Here's the drawing with two shaded views (mm, measured from the low corner). I have some questions. Coordinates: 2 decimals unless noted, no trailing zeros. Write each loop counter-clockwise with the first axis right and the second up, starting at its lowest first coordinate (ties: lowest second). Pieces come first, ordered by that corner, then holes. Notation, with made-up numbers: M 8,41 L 67,41 A29 ccw 67,62 Z; hole C 4.5,6.5 d1. An arc over 180 degrees is marked long. Use one line per item in the form item = value. Start each with the question number.
1. I want a section at C-C, the plane y = 17. List the corners of the cut face in (x, z) for me.
2. I want a section at D-D, the plane x = 48. List the corners of the cut face in (y, z) for me, plus the area to 3 significant figures.
3. I want a section at A-A, the plane z = 30. List the corners of the cut face in (x, y) for me.
4. I'm going to push flat-ended pins straight in: pin 1 Ø12 at (y, z) = (5.5, 13.5) entering from +X; pin 2 Ø12 at (y, z) = (16, 35.5) entering from +X; pin 3 Ø6 at (x, z) = (37.5, 19.5) entering from -Y; pin 4 Ø5 at (y, z) = (6.5, 27) entering from -X. Where does each tip first touch, or does it pass through?
5. I want a section at B-B, the plane x = 30. List the corners of the cut face in (y, z) for me.
6. Thinking about a two-plate mould opening in Z: for the marked faces 1, 2 and 3, which applies, released by +Z, released by -Z, zero draft, split by the parting line, or undercut?
7. Please list where these lines run through material, in increasing order: line 1 along X through (y, z) = (21.25, 30); line 2 along Z through (x, y) = (19, 10); line 3 along Z through (x, y) = (56.5, 2.5). Write a range as [from, to].
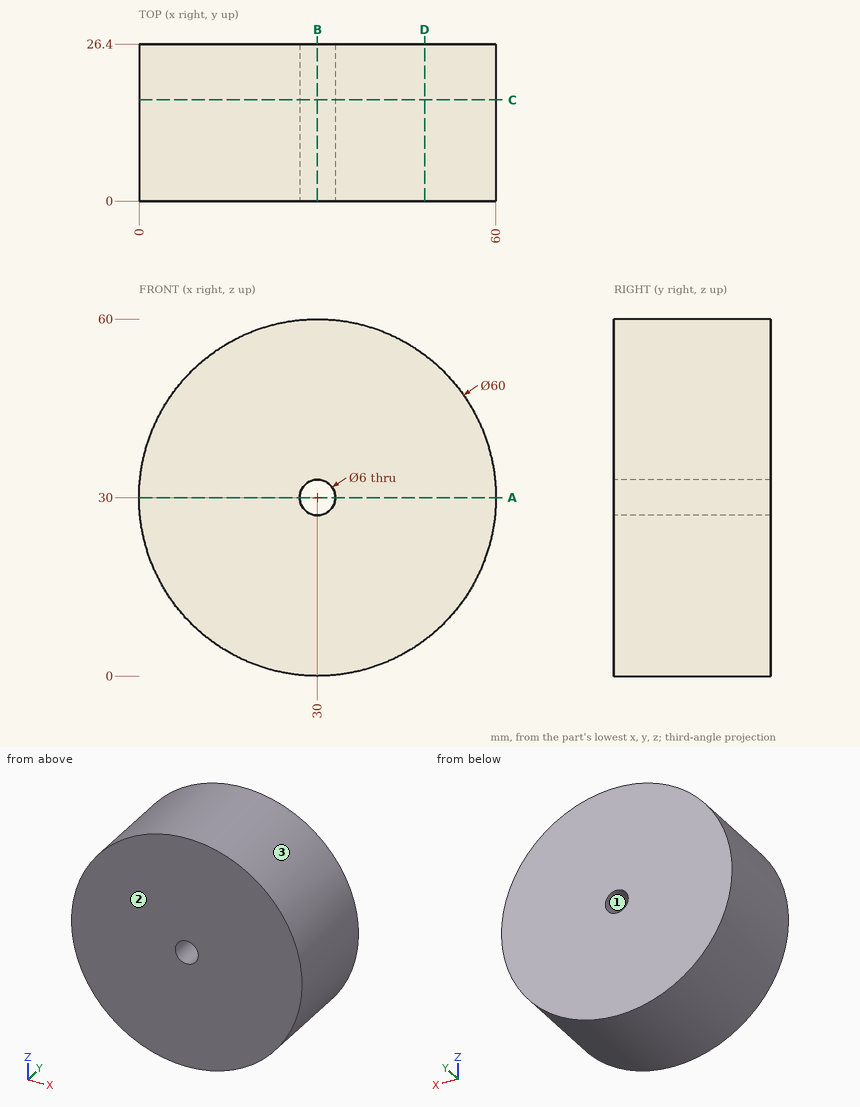
Answer list:
q1.outline = C 30,30 d60; hole C 30,30 d6
q2.outline = M 0,6 L 26.4,6 L 26.4,54 L 0,54 Z
q2.area = 1,270 mm²
q3.outline = M 0,0 L 27,0 L 27,26.4 L 0,26.4 Z; M 33,0 L 60,0 L 60,26.4 L 33,26.4 Z
q4.pin_1 = 58.1
q4.pin_2 = 60
q4.pin_3 = 0
q4.pin_4 = 0
q5.outline = M 0,0 L 26.4,0 L 26.4,27 L 0,27 Z; M 0,33 L 26.4,33 L 26.4,60 L 0,60 Z
q6.face_1 = undercut
q6.face_2 = zero draft
q6.face_3 = split by the parting line
q7.line_1 = [0, 27], [33, 60]
q7.line_2 = [2.09, 57.91]
q7.line_3 = [15.94, 44.06]
